Could you check a few things on this model? Use its own coordinates, in mm. Face numbers are marked on the shaded views. A direction names the side the tool comes from. Coordinates: 2 decimals unless noted, no trailing zeros. Order: outer loops, then holes, each group sorted by start corner. A loop starts at its lowest first (then second) coordinate and runs counter-clockwise, first axis right, second up. Notation, with made-up numbers: (8.25, 83) - (63.25, 83) arc R22 ccw to (63.25, 99) - close; hole circle Ø8 at (-12.5, 58.25). An arc over 180 degrees is marked (long way). One line per item, written item: value.
from build123d import *

# Parameters (mm, degrees)
SKETCH1_W           = 29
SKETCH1_H           = 13.5
BOSS_EXTRUDE1_DEPTH = 36
SKETCH2_W           = 26
SKETCH2_H           = 33
CUT_EXTRUDE1_DEPTH  = 12
CUT_EXTRUDE2_DEPTH  = 1.5
FILLET1_R           = 0.8


with BuildPart() as part:
    # Sketch1 → Boss-Extrude1 (new body)
    with BuildSketch(Plane.XY):
        with Locations((14.5, -6.75)):
            Rectangle(SKETCH1_W, SKETCH1_H)
    extrude(amount=BOSS_EXTRUDE1_DEPTH)

    # Sketch2 → Cut-Extrude1 (cut)
    with BuildSketch(Plane(origin=(0, 0, 0), x_dir=(1, 0, 0), z_dir=(0, 1, 0))):
        with Locations((14.5, -18)):
            Rectangle(SKETCH2_W, SKETCH2_H)
    extrude(amount=-CUT_EXTRUDE1_DEPTH, mode=Mode.SUBTRACT)

    # Sketch3 → Cut-Extrude2 (cut)
    with BuildSketch(Plane.XY.offset(36)):
        with BuildLine():
            Line((12, -1), (17, -1))
            ThreePointArc((17, -1), (19.5, -3.5), (17, -6))
            Line((17, -6), (12, -6))
            ThreePointArc((12, -6), (9.5, -3.5), (12, -1))
        make_face()
    extrude(amount=-CUT_EXTRUDE2_DEPTH, mode=Mode.SUBTRACT)

    # Fillet1
    fillet1_edges = [part.edges().sort_by_distance(p)[0] for p in [
        (29, -6.75, 36),
        (0, -6.75, 36),
        (29, -6.75, 0),
        (0, -6.75, 0),
    ]]
    fillet(fillet1_edges, radius=FILLET1_R)


solid = part.part
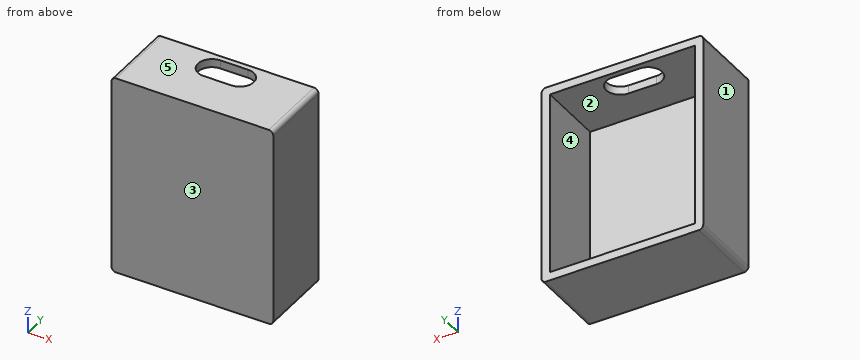
Item 1: I want a section at A-A on x = 14.25. Please give me the cut outline in (y, z), then the cut area to 3 significant figures.
Conclusion:
outline: (-13.5, 0) - (0, 0) - (0, 1.5) - (-12, 1.5) - (-12, 34.5) - (-6, 34.5) - (-6, 36) - (-13.5, 36) - close; (-1, 34.5) - (0, 34.5) - (0, 36) - (-1, 36) - close
area: 82.5 mm²
Item 2: I want a section at D-D on x = 22.25. Please give me the cut outline in (y, z), then the cut area to 3 significant figures.
Conclusion:
outline: (-13.5, 0) - (0, 0) - (0, 1.5) - (-12, 1.5) - (-12, 34.5) - (0, 34.5) - (0, 36) - (-13.5, 36) - close
area: 90.0 mm²
Item 3: I want a section at B-B on y = -8. Please give me the cut outline in (x, z), then the cut area to 3 significant figures.
Conclusion:
outline: (0, 0.8) arc R0.8 ccw to (0.8, 0) - (28.2, 0) arc R0.8 ccw to (29, 0.8) - (29, 35.2) arc R0.8 ccw to (28.2, 36) - (0.8, 36) arc R0.8 ccw to (0, 35.2) - close; hole (1.5, 1.5) - (27.5, 1.5) - (27.5, 34.5) - (1.5, 34.5) - close
area: 185 mm²
Item 4: Thinking about a two-plate mould opening in X: for the marked faces 1, 2 and 3, which applies, pulls with the +X half, pulls with the -X half, needs draft (parallel to the pull), parting line crosses it, or undercut?
Conclusion:
face 1: pulls with the -X half
face 2: undercut
face 3: needs draft
Item 5: If I drill on probe 1 along X at (y, z) = (-8.5, 12); probe 2 along Z at (x, y) = (19.25, -0.25); probe 3 along Y at (x, z) = (7, 6.5), over which ranges is the centre line in solid material (lowest first)?
Conclusion:
probe 1: 0 to 1.5, 27.5 to 29
probe 2: 0 to 1.5, 34.5 to 36
probe 3: -13.5 to -12
Item 6: I'm going to push flat-ended pins straight in: pin 1 Ø1 at (x, y) = (15.5, -2.5) entering from +Z; pin 2 Ø1.2 at (x, z) = (15.5, 35) entering from +Y. Where does each tip first touch, or does it pass through?
Conclusion:
pin 1: z = 1.5
pin 2: y = 0
Item 7: For the marked faces 4 and 5, which set-ups out of +Z, -Z, +X, -X, +Y, -Y let a thin tool reach every point of the face, with its end or its side?
Conclusion:
face 4: +Y
face 5: +Z, +X, -X, +Y, -Y
Item 8: I want a section at C-C on z = 24. Please give me the cut outline in (x, y), then the cut area to 3 significant figures.
Conclusion:
outline: (0, -13.5) - (29, -13.5) - (29, 0) - (27.5, 0) - (27.5, -12) - (1.5, -12) - (1.5, 0) - (0, 0) - close
area: 79.5 mm²
